from build123d import *

# Parameters (mm, degrees)
BASE_W                 = 120
BASE_H                 = 25
BASE_EXT_DEPTH         = 10
SKETCH3_R              = 5.5
LED_BOTTOM_CUT_DEPTH   = 63.469697574
LED_FOR_TOP_ROW_R      = 5.5
LED_TOP_CUT_DEPTH      = 65.13752525
SKETCH5_W              = 120
SKETCH5_H              = 25
SKETCH5_W_2            = 116
SKETCH5_H_2            = 21
WIRE_BOX_RIM_DEPTH     = 5
SKETCH6_W              = 6
SKETCH6_H              = 10
SUPPORT_SPACERS_DEPTH  = 5
SKETCH8_R              = 1.75
M3_SCREW_CUT_DEPTH     = 64.097147321
M3_NUT_CUT_DEPTH       = 3.5
WIRE_CUT_OUT_RX        = 2.5
WIRE_CUT_OUT_RY        = 2
WIRE_CUT_OUT_CUT_DEPTH = 2
FILLET1_R              = 1
FILLET2_R              = 1
FILLET3_R              = 2
FILLET4_R              = 2
FILLET5_R              = 2
FILLET6_R              = 2
FILLET7_R              = 8


with BuildPart() as part:
    # Base → Base EXT (new body)
    with BuildSketch(Plane(origin=(0, 0, 0), x_dir=(1, 0, 0), z_dir=(0, 1, 0))):
        Rectangle(BASE_W, BASE_H)
    extrude(amount=BASE_EXT_DEPTH)

    # Sketch3 → LED bottom CUT (cut, through all)
    with BuildSketch(Plane(origin=(0, 11.009339875, 0.963192432), x_dir=(1, 0, 0), z_dir=(0, 0.9961946980917455, 0.08715574274765836))):
        with Locations(Location((-45, 1.419123701, 0), (0, 0, 270))):
            Circle(SKETCH3_R)
        with Locations(Location((0, 1.419123701, 0), (0, 0, 270))):
            Circle(SKETCH3_R)
        with Locations(Location((45, 1.419123701, 0), (0, 0, 270))):
            Circle(SKETCH3_R)
    extrude(amount=-LED_BOTTOM_CUT_DEPTH, mode=Mode.SUBTRACT)

    # LED for Top Row → LED top CUT (cut, through all)
    with BuildSketch(Plane(origin=(0, 13.001715818, 6.062799655), x_dir=(1, 0, 0), z_dir=(0, 0.9063077870366496, 0.4226182617407003))):
        with Locations(Location((-23.903258736, 1.647335279, 0), (0, 0, 270))):
            Circle(LED_FOR_TOP_ROW_R)
        with Locations(Location((23.903258736, 1.647335279, 0), (0, 0, 270))):
            Circle(LED_FOR_TOP_ROW_R)
    extrude(amount=-LED_TOP_CUT_DEPTH, mode=Mode.SUBTRACT)

    # Sketch5 → Wire Box Rim (add)
    with BuildSketch(Plane(origin=(0, 10, 0), x_dir=(1, 0, 0), z_dir=(0, 1, 0))):
        Rectangle(SKETCH5_W, SKETCH5_H)
        Rectangle(SKETCH5_W_2, SKETCH5_H_2, mode=Mode.SUBTRACT)
    extrude(amount=WIRE_BOX_RIM_DEPTH)

    # Sketch6 → Support Spacers (add)
    with BuildSketch(Plane(origin=(0, 10, 0), x_dir=(1, 0, 0), z_dir=(0, 1, 0))):
        with Locations((-12, 0)):
            Rectangle(SKETCH6_W, SKETCH6_H)
        with Locations((12, 0)):
            Rectangle(SKETCH6_W, SKETCH6_H)
    extrude(amount=SUPPORT_SPACERS_DEPTH)

    # Sketch8 → M3 Screw CUT (cut, through all)
    with BuildSketch(Plane(origin=(0, 15, 0), x_dir=(1, 0, 0), z_dir=(0, 1, 0))):
        with Locations(Location((12, 0, 0), (0, 0, 270))):
            Circle(SKETCH8_R)
        with Locations(Location((-12, 0, 0), (0, 0, 90))):
            Circle(SKETCH8_R)
    extrude(amount=-M3_SCREW_CUT_DEPTH, mode=Mode.SUBTRACT)

    # M3 Nut → M3 Nut CUT (cut)
    with BuildSketch(Plane.XZ):
        Polygon((-12, 3.175426481), (-14.75, 1.58771324), (-14.75, -1.58771324), (-12, -3.175426481), (-9.25, -1.58771324), (-9.25, 1.58771324), align=None)
        Polygon((9.25, 1.58771324), (12, 3.175426481), (14.75, 1.58771324), (14.75, -1.58771324), (12, -3.175426481), (9.25, -1.58771324), align=None)
    extrude(amount=-M3_NUT_CUT_DEPTH, mode=Mode.SUBTRACT)

    # Wire cut out → Wire cut out CUT (cut)
    with BuildSketch(Plane(origin=(0, 0, -12.5), x_dir=(-1, 0, 0), z_dir=(0, 0, -1))):
        with Locations(Location((0, 15), (0, 0, 180))):
            Ellipse(WIRE_CUT_OUT_RX, WIRE_CUT_OUT_RY)
    extrude(amount=-WIRE_CUT_OUT_CUT_DEPTH, mode=Mode.SUBTRACT)

    # Fillet1
    fillet1_edges = [part.edges().sort_by_distance(p)[0] for p in [
        (2.5, 15, -11.5),
    ]]
    fillet(fillet1_edges, radius=FILLET1_R)

    # Fillet2
    fillet2_edges = [part.edges().sort_by_distance(p)[0] for p in [
        (-2.5, 15, -11.5),
    ]]
    fillet(fillet2_edges, radius=FILLET2_R)

    # Fillet3
    fillet3_edges = [part.edges().sort_by_distance(p)[0] for p in [
        (-60, 7.5, -12.5),
    ]]
    fillet(fillet3_edges, radius=FILLET3_R)

    # Fillet4
    fillet4_edges = [part.edges().sort_by_distance(p)[0] for p in [
        (60, 7.5, -12.5),
    ]]
    fillet(fillet4_edges, radius=FILLET4_R)

    # Fillet5
    fillet5_edges = [part.edges().sort_by_distance(p)[0] for p in [
        (60, 7.5, 12.5),
    ]]
    fillet(fillet5_edges, radius=FILLET5_R)

    # Fillet6
    fillet6_edges = [part.edges().sort_by_distance(p)[0] for p in [
        (-60, 7.5, 12.5),
    ]]
    fillet(fillet6_edges, radius=FILLET6_R)

    # Fillet7
    # the kernel refuses this fillet: 8 mm, written as the material it takes off along each edge
    with BuildSketch(Plane(origin=(78, 0, 12.5), x_dir=(0, 1, 0), z_dir=(-1, 0, 0))) as fillet7_piece_1:
        with BuildLine():
            CenterArc((FILLET7_R, FILLET7_R), FILLET7_R, 180, 90)
            Line((0, FILLET7_R), (0, 0))
            Line((0, 0), (FILLET7_R, 0))
        make_face()
    extrude(amount=156, mode=Mode.SUBTRACT)


solid = part.part
Verification items for the finished model (mm, model axes). A direction names the side the tool comes from. Give positions to 0.01 mm unless a question says otherwise; leave off trailing zeros. Loops run counter-clockwise (first coordinate to the right, second up) from the corner with the lowest first, then second, coordinate; pieces in that order, holes last.
1) Sectioned sample at B-B, the plane z = 0. Count the separate pieces of the cut face and the enclosed holes in it, then the cut area to 3 significant figures.
2) Set-up check for faces 1 (the cylindrical face through (-59.4, 7.4, -11.93)), 2 (the flat face through (58, 12, 0)), 3 (the flat face through (9.25, 2, 0)): record each of +Z, -Z, +X, -X, +Y, -Y from which the full face is reachable in a straight line by a thin tool's end or side.
3) Thickness scan on line 1 along X through (y, z) = (13.5, -2); line 2 along X through (y, z) = (11, 0); line 3 along X through (y, z) = (11, -9). Record the ranges inside material, lowest first.
4) Sectioned sample at A-A, the plane y = 11. Enter the section's corners in (x, z), then the cut area to 3 significant figures.
5) Draft check along X on faces 4 (the flat face through (-1, 7, -12.5)), 5 (the flat face through (12, 12, -5)), 6 (the flat face through (60, 7, 0)). Enter one of: pulls with the +X half, pulls with the -X half, needs draft (parallel to the pull), parting line crosses it, or undercut.
Answers:
1. separate pieces: 8
1. enclosed holes: 0
1. area: 623 mm2
2. face 1: -Z, -X, +Y, -Y
2. face 2: +Y
2. face 3: -Y
3. line 1: x = -60 to -58, -15 to -9, 9 to 15, 58 to 60
3. line 2: x = -60 to -58, -15 to -13.75, -10.25 to -9, 9 to 10.25, 13.75 to 15, 58 to 60
3. line 3: x = -60 to -58, 58 to 60
4. outline: (-60, -10.5) arc R2 ccw to (-58, -12.5) - (58, -12.5) arc R2 ccw to (60, -10.5) - (60, 10.5) arc R2 ccw to (58, 12.5) - (-58, 12.5) arc R2 ccw to (-60, 10.5) - close; (-15, -5) - (-9, -5) - (-9, 5) - (-15, 5) - close; (9, -5) - (15, -5) - (15, 5) - (9, 5) - close; hole (-58, -10.5) - (58, -10.5) - (58, 10.5) - (-58, 10.5) - close; hole circle Ø3.5 at (-12, 0); hole circle Ø3.5 at (12, 0)
4. area: 661 mm2
5. face 4: needs draft
5. face 5: undercut
5. face 6: pulls with the +X half
